The drawing under review shows one solid part. Ordinate dimensions are in mm from its lowest x, y, z. A direction names the side the tool comes from. Coordinates: 2 decimals unless noted, no trailing zeros. Loops run counter-clockwise (first coordinate to the right, second up) from the corner with the lowest first, then second, coordinate; pieces in that order, holes last. Notation, with made-up numbers: (44, 66) - (74, 66) arc R31 ccw to (74, 90) - close; hole circle Ø1 at (57, -23.5). An arc over 180 degrees is marked (long way). Use one line per item in the form item = value. Start each with the question number.
1. Add section B-B on x = 16.5. Give the boundary of the cut face in (y, z) (3 decimals).
2. For pin 1 Ø12 at (x, y) = (15, 49.5) entering from +Z; pin 2 Ø2 at (y, z) = (79, 22) entering from -X; pin 3 Ø3.5 at (x, z) = (10.033, 33.274) entering from -Y; pin 4 Ø4 at (x, z) = (4, 20) entering from -Y, all flat-tipped, find the tip position at first contact; note any pin that passes through.
3. To check wall thickness, follow probe 1 along Y at (x, z) = (13.75, 29.5); probe 2 along Z at (x, y) = (18.5, 62.5); probe 3 along Z at (x, y) = (15.75, 70.5). State the ranges of each line that lie inside material, in increasing order.
4. Add section D-D on z = 28. Give the boundary of the cut face in (x, y), and give its area (3 significant figures).
5. Machinability: for the marked faces 1, 2 and 3, which of the approach directions +Z, -Z, +X, -X, +Y, -Y give a long, thin tool a straight path to every point of the face, cutting with its end or side? Answer none if there is none.
6. Add section C-C on y = 79.5. Give the boundary of the cut face in (x, z), and give its area (3 significant figures).
7. Add section A-A on y = 8. Give the boundary of the cut face in (x, z).
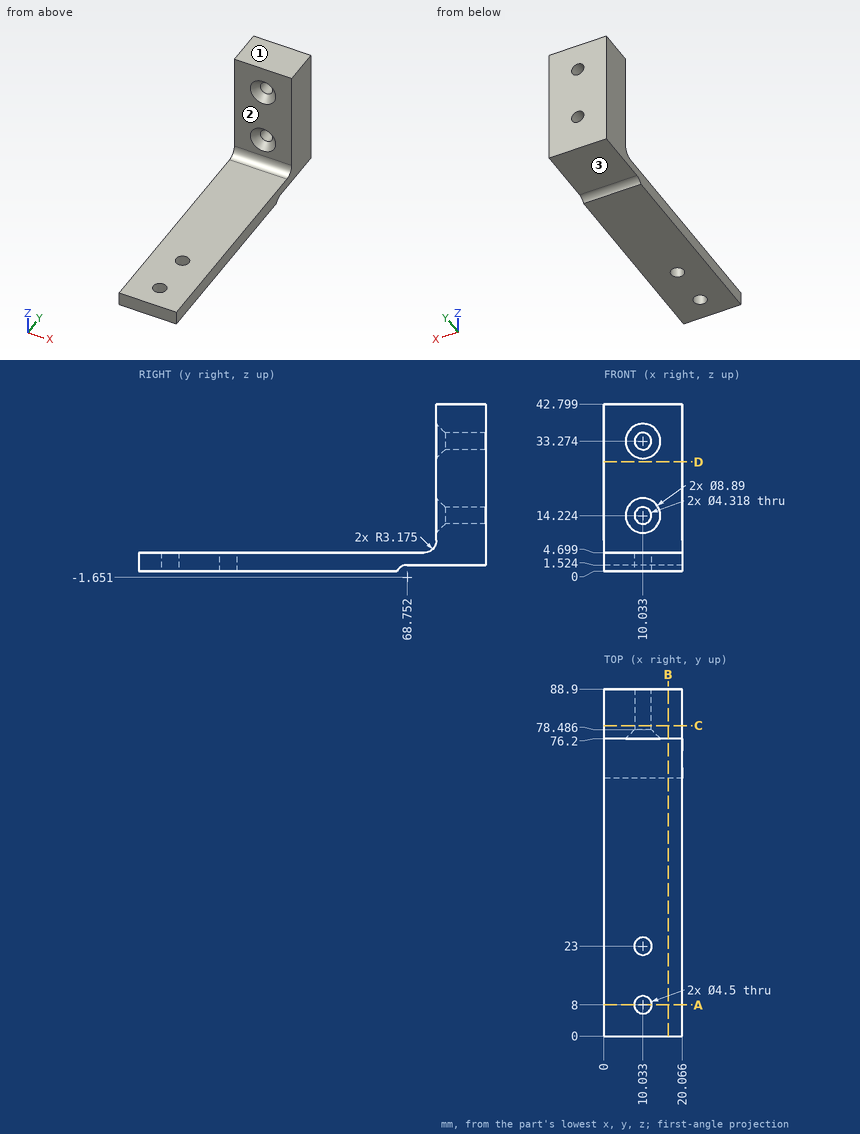
Conclusion:
q1.outline = (0, 0) - (66.04, 0) arc R3.175 cw to (68.752, 1.524) - (88.9, 1.524) - (88.9, 42.799) - (76.2, 42.799) - (76.2, 7.874) arc R3.175 cw to (73.025, 4.699) - (0, 4.699) - close
q2.pin_1 = 4.7
q2.pin_2 = 0
q2.pin_3 = through
q2.pin_4 = 76.2
q3.probe_1 = 76.2 to 88.9
q3.probe_2 = 0 to 4.7
q3.probe_3 = 1.52 to 4.7
q4.outline = (0, 76.2) - (20.07, 76.2) - (20.07, 88.9) - (0, 88.9) - close
q4.area = 255 mm^2
q5.face_1 = +Z, +X, -X, +Y, -Y
q5.face_2 = +Z, +X, -X, -Y
q5.face_3 = -Z, +X, -X, +Y
q6.outline = (0, 1.52) - (20.07, 1.52) - (20.07, 42.8) - (0, 42.8) - close; hole circle Ø4.32 at (10.03, 14.22); hole circle Ø4.32 at (10.03, 33.27)
q6.area = 799 mm^2
q7.outline = (0, 0) - (7.78, 0) - (7.78, 4.7) - (0, 4.7) - close; (12.28, 0) - (20.07, 0) - (20.07, 4.7) - (12.28, 4.7) - close
